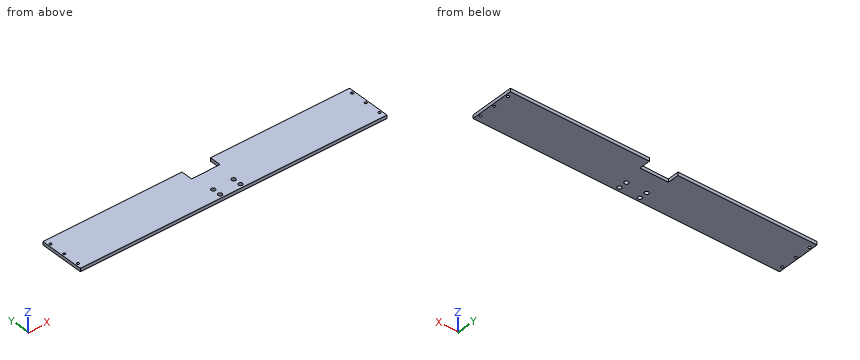
```python
from build123d import *

# Parameters (mm, degrees)
ESQUISSE1_W             = 752.95
ESQUISSE1_H             = 110
BOSS_EXTRU_1_DEPTH      = 8
ENL_V_MAT_EXTRU_1_REACH = 762.985
ESQUISSE2_R             = 5
ENL_V_MAT_EXTRU_2_REACH = 762.985
ESQUISSE3_R             = 3
ENL_V_MAT_EXTRU_3_REACH = 762.985
ESQUISSE4_W             = 70
ESQUISSE4_H             = 28


with BuildPart() as part:
    # Esquisse1 → Boss.-Extru.1 (new body)
    with BuildSketch(Plane.XY):
        with Locations((376.475, 55)):
            Rectangle(ESQUISSE1_W, ESQUISSE1_H)
    extrude(amount=BOSS_EXTRU_1_DEPTH)

    # Esquisse2 → Enlèv. mat.-Extru.1 (cut, up to next)
    with BuildSketch(Plane.XY.offset(8), mode=Mode.PRIVATE) as enl_v_mat_extru_1_sk1:
        with Locations((351.475, 30)):
            Circle(ESQUISSE2_R)
    enl_v_mat_extru_1_tool1 = extrude(enl_v_mat_extru_1_sk1.sketch, amount=-ENL_V_MAT_EXTRU_1_REACH, mode=Mode.PRIVATE) & part.part
    # Esquisse2 → Enlèv. mat.-Extru.1 (cut, up to next)
    with BuildSketch(Plane.XY.offset(8), mode=Mode.PRIVATE) as enl_v_mat_extru_1_sk2:
        with Locations((351.475, 10)):
            Circle(ESQUISSE2_R)
    enl_v_mat_extru_1_tool2 = extrude(enl_v_mat_extru_1_sk2.sketch, amount=-ENL_V_MAT_EXTRU_1_REACH, mode=Mode.PRIVATE) & part.part
    # Esquisse2 → Enlèv. mat.-Extru.1 (cut, up to next)
    with BuildSketch(Plane.XY.offset(8), mode=Mode.PRIVATE) as enl_v_mat_extru_1_sk3:
        with Locations(Location((401.475, 30, 0), (0, 0, 180))):
            Circle(ESQUISSE2_R)
    enl_v_mat_extru_1_tool3 = extrude(enl_v_mat_extru_1_sk3.sketch, amount=-ENL_V_MAT_EXTRU_1_REACH, mode=Mode.PRIVATE) & part.part
    # Esquisse2 → Enlèv. mat.-Extru.1 (cut, up to next)
    with BuildSketch(Plane.XY.offset(8), mode=Mode.PRIVATE) as enl_v_mat_extru_1_sk4:
        with Locations(Location((401.475, 10, 0), (0, 0, 180))):
            Circle(ESQUISSE2_R)
    enl_v_mat_extru_1_tool4 = extrude(enl_v_mat_extru_1_sk4.sketch, amount=-ENL_V_MAT_EXTRU_1_REACH, mode=Mode.PRIVATE) & part.part
    add(enl_v_mat_extru_1_tool1.solids().sort_by_distance((351.475, 30, 8))[0], mode=Mode.SUBTRACT)
    add(enl_v_mat_extru_1_tool2.solids().sort_by_distance((351.475, 10, 8))[0], mode=Mode.SUBTRACT)
    add(enl_v_mat_extru_1_tool3.solids().sort_by_distance((401.475, 30, 8))[0], mode=Mode.SUBTRACT)
    add(enl_v_mat_extru_1_tool4.solids().sort_by_distance((401.475, 10, 8))[0], mode=Mode.SUBTRACT)

    # Esquisse3 → Enlèv. mat.-Extru.2 (cut, up to next)
    with BuildSketch(Plane.XY.offset(8), mode=Mode.PRIVATE) as enl_v_mat_extru_2_sk1:
        with Locations((6, 95)):
            Circle(ESQUISSE3_R)
    enl_v_mat_extru_2_tool1 = extrude(enl_v_mat_extru_2_sk1.sketch, amount=-ENL_V_MAT_EXTRU_2_REACH, mode=Mode.PRIVATE) & part.part
    # Esquisse3 → Enlèv. mat.-Extru.2 (cut, up to next)
    with BuildSketch(Plane.XY.offset(8), mode=Mode.PRIVATE) as enl_v_mat_extru_2_sk2:
        with Locations((6, 55)):
            Circle(ESQUISSE3_R)
    enl_v_mat_extru_2_tool2 = extrude(enl_v_mat_extru_2_sk2.sketch, amount=-ENL_V_MAT_EXTRU_2_REACH, mode=Mode.PRIVATE) & part.part
    # Esquisse3 → Enlèv. mat.-Extru.2 (cut, up to next)
    with BuildSketch(Plane.XY.offset(8), mode=Mode.PRIVATE) as enl_v_mat_extru_2_sk3:
        with Locations((6, 15)):
            Circle(ESQUISSE3_R)
    enl_v_mat_extru_2_tool3 = extrude(enl_v_mat_extru_2_sk3.sketch, amount=-ENL_V_MAT_EXTRU_2_REACH, mode=Mode.PRIVATE) & part.part
    # Esquisse3 → Enlèv. mat.-Extru.2 (cut, up to next)
    with BuildSketch(Plane.XY.offset(8), mode=Mode.PRIVATE) as enl_v_mat_extru_2_sk4:
        with Locations(Location((746.95, 15, 0), (0, 0, 180))):
            Circle(ESQUISSE3_R)
    enl_v_mat_extru_2_tool4 = extrude(enl_v_mat_extru_2_sk4.sketch, amount=-ENL_V_MAT_EXTRU_2_REACH, mode=Mode.PRIVATE) & part.part
    # Esquisse3 → Enlèv. mat.-Extru.2 (cut, up to next)
    with BuildSketch(Plane.XY.offset(8), mode=Mode.PRIVATE) as enl_v_mat_extru_2_sk5:
        with Locations(Location((746.95, 55, 0), (0, 0, 180))):
            Circle(ESQUISSE3_R)
    enl_v_mat_extru_2_tool5 = extrude(enl_v_mat_extru_2_sk5.sketch, amount=-ENL_V_MAT_EXTRU_2_REACH, mode=Mode.PRIVATE) & part.part
    # Esquisse3 → Enlèv. mat.-Extru.2 (cut, up to next)
    with BuildSketch(Plane.XY.offset(8), mode=Mode.PRIVATE) as enl_v_mat_extru_2_sk6:
        with Locations(Location((746.95, 95, 0), (0, 0, 180))):
            Circle(ESQUISSE3_R)
    enl_v_mat_extru_2_tool6 = extrude(enl_v_mat_extru_2_sk6.sketch, amount=-ENL_V_MAT_EXTRU_2_REACH, mode=Mode.PRIVATE) & part.part
    add(enl_v_mat_extru_2_tool1.solids().sort_by_distance((6, 95, 8))[0], mode=Mode.SUBTRACT)
    add(enl_v_mat_extru_2_tool2.solids().sort_by_distance((6, 55, 8))[0], mode=Mode.SUBTRACT)
    add(enl_v_mat_extru_2_tool3.solids().sort_by_distance((6, 15, 8))[0], mode=Mode.SUBTRACT)
    add(enl_v_mat_extru_2_tool4.solids().sort_by_distance((746.95, 15, 8))[0], mode=Mode.SUBTRACT)
    add(enl_v_mat_extru_2_tool5.solids().sort_by_distance((746.95, 55, 8))[0], mode=Mode.SUBTRACT)
    add(enl_v_mat_extru_2_tool6.solids().sort_by_distance((746.95, 95, 8))[0], mode=Mode.SUBTRACT)

    # Esquisse4 → Enlèv. mat.-Extru.3 (cut, up to next)
    with BuildSketch(Plane.XY.offset(8), mode=Mode.PRIVATE) as enl_v_mat_extru_3_sk1:
        with Locations((376.475, 96)):
            Rectangle(ESQUISSE4_W, ESQUISSE4_H)
    enl_v_mat_extru_3_tool1 = extrude(enl_v_mat_extru_3_sk1.sketch, amount=-ENL_V_MAT_EXTRU_3_REACH, mode=Mode.PRIVATE) & part.part
    add(enl_v_mat_extru_3_tool1.solids().sort_by_distance((376.475, 96, 8))[0], mode=Mode.SUBTRACT)


solid = part.part
```
Model file for the job. Use its own axes, mm. Round coordinates to 2 decimals unless told otherwise and drop trailing zeros. Put each result on its own line as item: value. Start each with the question number.
Item 1: Drill centre lines: line 1 along Y through (x, z) = (6, 2); line 2 along X through (y, z) = (100.5, 3.5) (3 decimals); line 3 along X through (y, z) = (17, 5.75). Where is each one in solid material? Low to high.
Item 2: Drop flat-ended pins along their axis: P1, Ø1.5, axis at x = 412, y = 85, coming from the -Z side; P2, Ø5, axis at x = 6, y = 15, coming from the +Z side; P3, Ø2.5, axis at x = 384.5, z = 4.5, coming from the +Y side. Give the stop position or say it passes through.
Item 3: Cut at A-A (z = 4). Give the number of separate pieces and of enclosed holes in the cut face, then the cut area to 3 significant figures.
Answer block:
1. line 1: 0 to 12, 18 to 52, 58 to 92, 98 to 110
1. line 2: 0 to 341.475, 411.475 to 752.95
1. line 3: 0 to 3.76, 8.24 to 744.71, 749.19 to 752.95
2. P1: z = 0
2. P2: through
2. P3: y = 82
3. separate pieces: 1
3. enclosed holes: 10
3. area: 80,400 mm2
